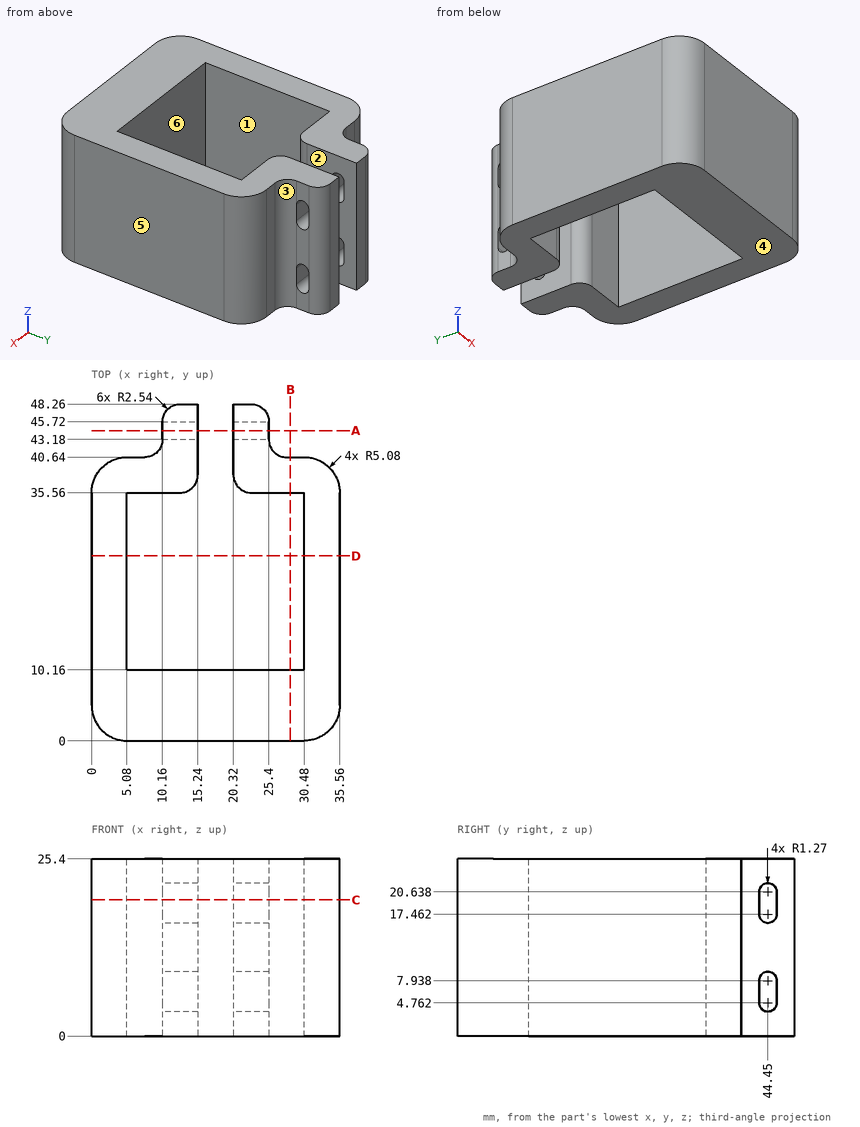
Drawing for the job (mm, zero at the part's lowest x, y, z). A direction names the side the tool comes from. Round coordinates to 2 decimals unless told otherwise and drop trailing zeros. Write each loop counter-clockwise with the first axis right and the second up, starting at its lowest first coordinate (ties: lowest second). Pieces come first, ordered by that corner, then holes. Notation, with made-up numbers: (62, -11.75) - (110, -11.75) arc R31 cw to (110, 21.25) - close; hole circle Ø1 at (47.25, 23). An arc over 180 degrees is marked (long way). Return JSON: item names as keys, results as strings. Group by question number.
Item 1: 3-axis set-ups, long thin cutter, end or side, ignore diameter. For the marked faces 1, 2 and 3: which of +Z, -Z, +X, -X, +Y, -Y reach the whole face in a straight line?
Item 2: Probe probe 1 along Y at (x, z) = (29, 21.25); probe 2 along X at (y, z) = (14.5, 9.25); probe 3 along Y at (x, z) = (22.5, 7.5) (1 decimal). List the from-to ranges inside material, lowest first.
Item 3: Band-saw the part on A-A on y = 44.45. List the corners of the cut face in (x, z), plus the area to 3 significant figures.
Item 4: Band-saw the part on D-D on y = 26.5. List the corners of the cut face in (x, z), plus the area to 3 significant figures.
Item 5: Mould opens along X. For the marked faces 4, 5 and 6 say: +X half, -X half, draft (parallel to the pull), parting line (faces both ways), or undercut.
Item 6: Band-saw the part on C-C on z = 19.5. State how many separate pieces and enclosed holes the cut face has, plus the area to 3 significant figures.
Item 7: Band-saw the part on B-B on x = 28.5. List the corners of the cut face in (y, z).
Item 8: Flat gauge pins, fed straight in: pin 1 Ø1.3 at (x, z) = (29.5, 6.5) entering from +Y; pin 2 Ø2 at (y, z) = (44, 3) entering from -X; pin 3 Ø5 at (y, z) = (42.5, 18) entering from -X. Where does each tip first touch, or does it go through?
Resolved:
{
 "1": {"face 1": "+Z, -Z", "face 2": "+Z, -Z, +Y", "face 3": "+Z, -Z, +X, +Y"},
 "2": {"probe 1": "y = 0 to 10.16, 35.56 to 40.64", "probe 2": "x = 0 to 5.08, 30.48 to 35.56", "probe 3": "y = 0 to 10.2, 35.6 to 43.2, 45.7 to 48.3"},
 "3": {"outline": "(10.16, 0) - (15.24, 0) - (15.24, 3.49) - (10.16, 3.49) - close; (10.16, 9.21) - (15.24, 9.21) - (15.24, 16.19) - (10.16, 16.19) - close; (10.16, 21.91) - (15.24, 21.91) - (15.24, 25.4) - (10.16, 25.4) - close; (20.32, 0) - (25.4, 0) - (25.4, 3.49) - (20.32, 3.49) - close; (20.32, 9.21) - (25.4, 9.21) - (25.4, 16.19) - (20.32, 16.19) - close; (20.32, 21.91) - (25.4, 21.91) - (25.4, 25.4) - (20.32, 25.4) - close", "area": "142 mm²"},
 "4": {"outline": "(0, 0) - (5.08, 0) - (5.08, 25.4) - (0, 25.4) - close; (30.48, 0) - (35.56, 0) - (35.56, 25.4) - (30.48, 25.4) - close", "area": "258 mm²"},
 "5": {"face 4": "draft", "face 5": "+X half", "face 6": "undercut"},
 "6": {"separate pieces": "3", "enclosed holes": "0", "area": "801 mm²"},
 "7": {"outline": "(0, 0) - (10.16, 0) - (10.16, 25.4) - (0, 25.4) - close; (35.56, 0) - (40.64, 0) - (40.64, 25.4) - (35.56, 25.4) - close"},
 "8": {"pin 1": "stops at y = 40.64", "pin 2": "stops at x = 10.15", "pin 3": "stops at x = 2.61"}
}
